Could you check a few things on this model? Use its own coordinates, in mm. Round coordinates to 2 decimals unless told otherwise and drop trailing zeros. Order: outer loops, then holes, each group sorted by start corner. A loop starts at its lowest first (then second) coordinate and runs counter-clockwise, first axis right, second up.
Autodesk Inventor part; units mm, degrees
ref_plane "YZ Plane" through (0, 0, 0) normal (1, 0, 0) x (0, 1, 0)
ref_plane "XZ Plane" through (0, 0, 0) normal (0, 1, 0) x (-1, 0, 0)
ref_plane "XY Plane" through (0, 0, 0) normal (0, 0, 1) x (1, 0, 0)
sketch "Sketch1" plane through (0, 0, 0) normal (0, 0, 1) x (1, 0, 0)
  line L0 (-12.1708, 16.0073) -> (13.2292, 16.0073)
  line L1 (13.2292, 16.0073) -> (13.2292, -34.7927)
  line L2 (13.2292, -34.7927) -> (-12.1708, -34.7927)
  line L3 (-12.1708, -34.7927) -> (-12.1708, 16.0073)
  line L4 (11.9592, 14.7373) -> (-10.9008, 14.7373)
  line L5 (-10.9008, 14.7373) -> (-10.9008, -33.5227)
  line L6 (-10.9008, -33.5227) -> (11.9592, -33.5227)
  line L7 (11.9592, -33.5227) -> (11.9592, 14.7373)
  point P0 (0, 0)
  dimension "d0" = 25.4
  dimension "d1" = 50.8
  dimension "d2" = 1.27
extrude "Extrusion1" add sketch "Sketch1" along normal blind 304.8
sketch "Sketch2" plane through (-12.1708, 16.0073, 0) normal (0, 1, 0) x (1, 0, 0)
  circle A0 centre (12.7, -12.7) radius 1.7272
  line L0 (25.4, 0) -> (0, 0)
  line L1 (0, 0) -> (0, -304.8)
  point P0 (12.1708, 0)
  dimension "d5" = 3.4544
  dimension "d6" = 12.7
  dimension "d7" = 12.7
extrude "Extrusion2" cut sketch "Sketch2" against normal through all
pattern_linear "Rectangular Pattern1" count 12 spacing 25.4 along (0, 0, 1) of "Extrusion2"
sketch "Sketch5" plane through (13.2292, -34.7927, 0) normal (1, 0, 0) x (0, 0, -1)
  line L0 (-304.8, 50.8) -> (-304.8, 0)
  line L1 (-304.8, 25.4) -> (117.859, 25.4) construction
  circle A0 centre (-279.4, 25.4) radius 14.2875
  circle A1 centre (-25.4, 25.4) radius 14.2875
  point P0 (0, 34.7927)
  dimension "d26" = 28.575
  dimension "d27" = 254
  dimension "d28" = 25.4
extrude "Extrusion5" cut sketch "Sketch5" against normal through all
equation "\"d3\" = d13"
equation "\"d13\" = 304.8"
properties part number "VerseFrame 12in for BS"
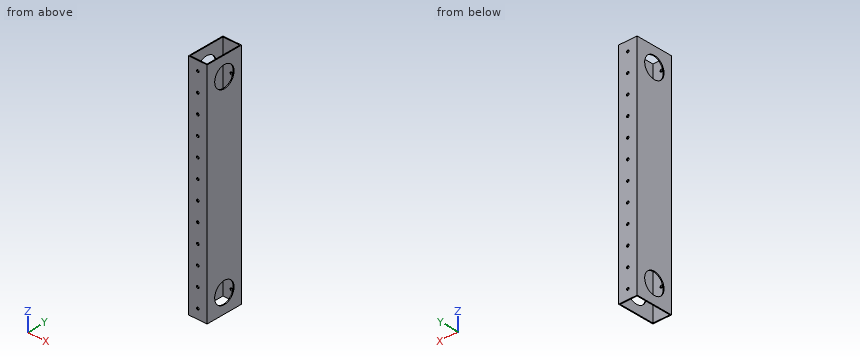
Q1. Imagine slicing it at B-B, the plane x = 6.25. Please give me the cut outline in (y, z), then the cut area to 3 significant figures.
Q2. Imagine slicing it at D-D, the plane z = 19.5. Please give me the cut outline in (x, y), then the cut area to 3 significant figures.
Q3. I need wall thicknesses on L1, parallel to Y at x = -3.25, z = 200; L2, parallel to X at y = -13.5, z = 88; L3, parallel to X at y = 15.3, z = 190.5. Which ranges of each line are inside material? Lowest first, please.
Q4. Imagine slicing it at C-C, the plane y = -30.5. Please give me the cut outline in (x, z).
Q5. Imagine slicing it at A-A, the plane z = 230.5. Please give me the cut outline in (x, y).
Filled in:
1. outline: (-34.79, 0) - (-33.52, 0) - (-33.52, 304.8) - (-34.79, 304.8) - close; (14.74, 0) - (16.01, 0) - (16.01, 304.8) - (14.74, 304.8) - close
1. area: 774 mm2
2. outline: (-12.17, -34.79) - (13.23, -34.79) - (13.23, -22.41) - (11.96, -22.41) - (11.96, -33.52) - (-10.9, -33.52) - (-10.9, -22.41) - (-12.17, -22.41) - close; (-12.17, 3.62) - (-10.9, 3.62) - (-10.9, 14.74) - (11.96, 14.74) - (11.96, 3.62) - (13.23, 3.62) - (13.23, 16.01) - (-12.17, 16.01) - close
2. area: 121 mm2
3. L1: y = -34.79 to -33.52, 14.74 to 16.01
3. L2: x = -12.17 to -10.9, 11.96 to 13.23
3. L3: x = -12.17 to -1.2, 2.26 to 13.23
4. outline: (-12.17, 0) - (-10.9, 0) - (-10.9, 304.8) - (-12.17, 304.8) - close; (11.96, 0) - (13.23, 0) - (13.23, 304.8) - (11.96, 304.8) - close
5. outline: (-12.17, -34.79) - (13.23, -34.79) - (13.23, 16.01) - (-12.17, 16.01) - close; hole (-10.9, -33.52) - (11.96, -33.52) - (11.96, 14.74) - (-10.9, 14.74) - close
